Read the model definition and answer for the solid it produces. Units are mm, in the model's axes. A direction names the side the tool comes from. Round coordinates to 2 decimals unless told otherwise and drop trailing zeros. Order: outer loops, then holes, each group sorted by start corner. A loop starts at its lowest first (then second) coordinate and runs counter-clockwise, first axis right, second up. Notation, with made-up numbers: (-39, 79) - (-11, 79) arc R15 ccw to (-11, 93) - close; hole circle Ø7 at (-32, -19.75). An arc over 180 degrees is marked (long way). Put each result on its own line as item: value. Start each with the question number.
Q1. Section D-D on x = 34 is taken. Give the vertices of the cut face in (y, z).
Q2. Section C-C on z = -9 is taken. Give the vertices of the cut face in (x, y) (3 decimals).
Q3. Which of the six approach directions +Z, -Z, +X, -X, +Y, -Y give full straight-line access (tool end or side, diameter ignored) to faces 5 (the face through (24.15, 400.62, 12.1)), 6 (the face through (1, 356, 0)), 7 (the face through (25.4, 439, 24)), 8 (the face through (-25.4, 439, 24)), 9 (the face through (-22.86, 398, 15))?
Q4. Section B-B on y = 451 is taken. Give the vertices of the cut face in (x, z), then the cut area to 3 significant figures.
Q5. Each of these flat-tipped pins is pushed along its axis until it touches: pin 1 Ø15 at (x, y) = (16, 358.5) entering from +Z; pin 2 Ø12.5 at (y, z) = (432.5, 22.5) entering from -X; pin 3 Ø1.5 at (x, y) = (24, 434) entering from -Z. Where does it stop, or does it pass through?
Q6. For a pull along Y with two mould halves and no side action, classify faces 1 (the face through (-1.707, 364.957, -6.439)), 2 (the face through (98.188, 370, -1)), 3 (the face through (1, 330.2, -6)), 4 (the face through (-3.16, 440.35, 24.98)) as pulls with the +Y half, pulls with the -Y half, needs draft (parallel to the pull), parting line crosses it, or undercut.
Q7. Find the intervals of material crossed by line 1 along Y through (x, z) = (0, 26.75); line 2 along X through (y, z) = (398.5, 19); line 3 along Y through (x, z) = (-79.5, -3.5), in increasing order. Write a range as from..to.
Q8. Section A-A on x = 0 is taken. Give the vertices of the cut face in (y, z).
Autodesk Inventor part; units mm, degrees
ref_plane "YZ Plane" through (0, 0, 0) normal (1, 0, 0) x (0, 1, 0)
ref_plane "XZ Plane" through (0, 0, 0) normal (0, 1, 0) x (-1, 0, 0)
ref_plane "XY Plane" through (0, 0, 0) normal (0, 0, 1) x (1, 0, 0)
sketch "Sketch2" plane through (0, 0, 0) normal (0, 0, 1) x (1, 0, 0)
  circle A0 centre (0, 0) radius 406.4
  line L0 (-704.85, -381) -> (704.85, -381)
  line L1 (704.85, -381) -> (704.85, 381)
  line L2 (-704.85, 381) -> (-704.85, -381)
  line L3 (-704.85, -381) -> (704.85, 381) construction
  line L4 (704.85, -381) -> (-704.85, 381) construction
  line L5 (0, 381) -> (-98.1878, 381)
  line L6 (0, 394.3604) -> (-98.1878, 394.3604)
  line L7 (-98.1878, 394.3604) -> (-98.1878, 381)
  line L8 (0, 394.3604) -> (98.1878, 394.3604)
  line L9 (98.1878, 394.3604) -> (98.1878, 381)
  line L10 (-98.1878, 381) -> (98.1878, 381)
  line L11 (-98.1878, 381) -> (98.1878, 381)
  line L12 (-98.1878, 394.3604) -> (98.1878, 394.3604)
  line L13 (98.1878, 394.3604) -> (98.1878, 381)
  line L14 (-98.1878, 394.3604) -> (-98.1878, 381)
  line L15 (-141.4212, 381) -> (-704.85, 381)
  line L16 (704.85, 381) -> (141.4212, 381)
  line L17 (98.1878, 381) -> (-98.1878, 381)
  dimension "d0" = 812.8
  dimension "d1" = 1409.7
  dimension "d2" = 762
  dimension "d9" = 394.3604
extrude "Extrusion1" add sketch "Sketch2" along normal blind 31.242 contours L9 L10 L5 L7 L6 L8
sketch "Sketch4" plane through (0, 0, 31.242) normal (0, 0, 1) x (1, 0, 0)
  circle A0 centre (0, 0) radius 406.4
  line L0 (98.1878, 394.3604) -> (-98.1878, 394.3604)
  circle A1 centre (0, 454.5584) radius 14.5542
  line L1 (25.4, 394.3604) -> (-25.4, 394.3604)
  line L2 (-25.4, 394.3604) -> (-25.4, 483.2604)
  line L3 (-25.4, 483.2604) -> (25.4, 483.2604)
  line L4 (25.4, 483.2604) -> (25.4, 394.3604)
  line L5 (0, 0) -> (0, 517.5127)
  arc A2 (25.4, 410.5643) -> (-25.4, 410.5643) centre (0, 454.5584) ccw
  line L6 (-98.1878, 381) -> (98.1878, 381)
  dimension "d10" = 812.8
  dimension "d12" = 60.198
  dimension "d13" = 29.1084
  dimension "d14" = 50.8
  dimension "d15" = 88.9
  dimension "d16" = 25.4
  dimension "d27" = 13.3604
  dimension "d28" = 50.8
extrude "Extrusion2" add sketch "Sketch4" against normal blind 12.7 contours L4 L0 L5 A0 | A0 L5 A1 L3 L4 | L2 L3 L5 A1 A0 | A0 L5 L0 L2
sketch "Sketch7" plane through (0, 0, 0) normal (0, 0, -1) x (-1, 0, 0)
  line L0 (98.1878, 394.3604) -> (98.1878, 381)
  line L1 (98.1878, 394.3604) -> (-98.1878, 394.3604)
  line L2 (-98.1878, 394.3604) -> (-98.1878, 330.2)
  line L3 (-98.1878, 330.2) -> (98.1878, 330.2)
  line L4 (98.1878, 330.2) -> (98.1878, 394.3604)
  line L5 (98.1878, 381) -> (-98.1878, 381)
  point P0 (0, 0)
  dimension "d23" = 50.8
  dimension "d24" = 64.1604
extrude "Extrusion5" add sketch "Sketch7" along normal blind 12.7
sketch "Sketch8" plane through (0, 0, -12.7) normal (0, 0, -1) x (-1, 0, 0)
  line L0 (98.1878, 394.3604) -> (-98.1878, 394.3604)
  circle A0 centre (0, 362.2802) radius 3.175
  point P0 (0, 0)
  dimension "d31" = 6.35
extrude "Extrusion6" cut sketch "Sketch8" against normal blind 12.7
thread "Thread1"
sketch "Sketch9" plane through (-25.4, 394.3604, 31.242) normal (-1, 0, 0) x (0, 0, 1)
  line L0 (0, 88.9) -> (-12.7, 88.9)
  line L1 (-12.7, 88.9) -> (-12.7, 0)
  line L2 (-12.7, 12.7) -> (-12.7, 0)
  line L3 (-12.7, 0) -> (-25.4, 0)
  line L4 (-43.942, 0) -> (0, 0)
  line L5 (-25.4, 0) -> (-12.7, 12.7)
  point P0 (-31.242, -394.3604)
  dimension "d36" = 12.7
  dimension "d37" = 45
extrude "Extrusion7" add sketch "Sketch9" against normal blind 2.54
sketch "Sketch10" plane through (25.4, 394.3604, 31.242) normal (1, 0, 0) x (0, 0, -1)
  line L0 (25.4, 0) -> (12.7, 0)
  line L1 (25.4, 0) -> (12.7, 12.7)
  line L2 (12.7, 0) -> (12.7, 12.7)
  line L3 (12.7, 12.7) -> (25.4, 0)
  line L4 (25.4, 0) -> (12.7, 0)
  point P0 (31.242, -394.3604)
extrude "Extrusion8" add sketch "Sketch10" against normal blind 2.54
properties part number "NewNewMechanism"
Findings:
1. outline: (330.2, -12.7) - (394.36, -12.7) - (394.36, 31.24) - (381, 31.24) - (381, 0) - (330.2, 0) - close
2. outline: (-98.188, 330.2) - (98.188, 330.2) - (98.188, 394.36) - (-98.188, 394.36) - close; hole circle Ø6.35 at (0, 362.28)
3. face 5: -Z, +X, -X, +Y
3. face 6: +Z, +X, -X, -Y
3. face 7: +Z, -Z, +X, +Y
3. face 8: +Z, -Z, -X, +Y
3. face 9: -Z, +Y
4. outline: (-25.4, 18.54) - (-14.11, 18.54) - (-14.11, 31.24) - (-25.4, 31.24) - close; (14.11, 18.54) - (25.4, 18.54) - (25.4, 31.24) - (14.11, 31.24) - close
4. area: 287 mm2
5. pin 1: z = 0
5. pin 2: x = -25.4
5. pin 3: z = 18.54
6. face 1: undercut
6. face 2: needs draft
6. face 3: pulls with the -Y half
6. face 4: undercut
7. line 1: 381..440, 469.11..483.26
7. line 2: -25.4..25.4
7. line 3: 330.2..394.36
8. outline: (330.2, -12.7) - (359.11, -12.7) - (359.11, 0) - (330.2, 0) - close; (365.46, -12.7) - (394.36, -12.7) - (394.36, 18.54) - (440, 18.54) - (440, 31.24) - (381, 31.24) - (381, 0) - (365.46, 0) - close; (469.11, 18.54) - (483.26, 18.54) - (483.26, 31.24) - (469.11, 31.24) - close
